from build123d import *

# Parameters (mm, degrees)
BOSS_EXTRUDE1_DEPTH = 25
SKETCH5_R           = 5
CUT_EXTRUDE1_DEPTH  = 5000
SKETCH6_R           = 5
CUT_EXTRUDE2_DEPTH  = 5000
FILLET2_R           = 10


with BuildPart() as part:
    # Sketch4 → Boss-Extrude1 (new body)
    with BuildSketch(Plane.XY):
        with BuildLine():
            ThreePointArc((0, -25), (-77.42819254, 7.07180746), (-109.5, 84.5))
            Line((-109.5, 84.5), (-109.5, -25))
            Line((-109.5, -25), (0, -25))
        make_face()
        with BuildLine():
            ThreePointArc((84.5, 84.5), (59.75052301, 24.74947699), (0, 0))
            ThreePointArc((0, 0), (-59.75052301, 24.74947699), (-84.5, 84.5))
            Line((-84.5, 84.5), (-109.5, 84.5))
            ThreePointArc((-109.5, 84.5), (-77.42819254, 7.07180746), (0, -25))
            ThreePointArc((0, -25), (77.42819254, 7.07180746), (109.5, 84.5))
            Line((109.5, 84.5), (84.5, 84.5))
        make_face()
        with BuildLine():
            Line((109.5, -25), (109.5, 84.5))
            ThreePointArc((109.5, 84.5), (77.42819254, 7.07180746), (0, -25))
            Line((0, -25), (109.5, -25))
        make_face()
    extrude(amount=BOSS_EXTRUDE1_DEPTH)

    # Sketch5 → Cut-Extrude1 (cut)
    with BuildSketch(Plane(origin=(0, 84.5, 0), x_dir=(1, 0, 0), z_dir=(0, 1, 0))):
        with Locations((-97, -12.5)):
            Circle(SKETCH5_R)
        with Locations((97, -12.5)):
            Circle(SKETCH5_R)
    extrude(amount=-CUT_EXTRUDE1_DEPTH, mode=Mode.SUBTRACT)

    # Sketch6 → Cut-Extrude2 (cut)
    with BuildSketch(Plane.XY.offset(25)):
        with Locations((-76.015, -4)):
            Circle(SKETCH6_R)
        with Locations((76.015, -4)):
            Circle(SKETCH6_R)
    extrude(amount=-CUT_EXTRUDE2_DEPTH, mode=Mode.SUBTRACT)

    # Fillet2
    fillet2_edges = [part.edges().sort_by_distance(p)[0] for p in [
        (109.5, 29.75, 25),
        (-109.5, 29.75, 25),
        (-109.5, 29.75, 0),
        (109.5, 29.75, 0),
    ]]
    fillet(fillet2_edges, radius=FILLET2_R)


solid = part.part
Could you check a few things on this model? Use its own coordinates, in mm. Give positions to 0.01 mm unless a question says otherwise; leave off trailing zeros. Order: outer loops, then holes, each group sorted by start corner. A loop starts at its lowest first (then second) coordinate and runs counter-clockwise, first axis right, second up.
1. Thinking about a two-plate mould opening in Z: for faces 1 (the flat face through (-1, -6, 0)), 2 (the flat face through (-109.5, 31, 12)), 3 (the cylindrical face through (101.619, 30.516, 14.415)), which applies, +Z half, -Z half, draft (parallel to the pull), parting line (faces both ways), or undercut?
Answers below:
face 1: -Z half
face 2: draft
face 3: undercut
2. Suppose I cut it at D-D (y = 42.5). Write out the boundary of the cut face in (x, z).
Answers below:
outline: (-109.5, 10) arc R10 ccw to (-99.5, 0) - (-73.32, 0) - (-73.32, 25) - (-99.5, 25) arc R10 ccw to (-109.5, 15) - close; (73.32, 0) - (99.5, 0) arc R10 ccw to (109.5, 10) - (109.5, 15) arc R10 ccw to (99.5, 25) - (73.32, 25) - close; hole circle Ø10 at (-97, 12.5); hole circle Ø10 at (97, 12.5)
3. I need wall thicknesses on L1, parallel to Z at x = 97, y = 27; L2, parallel to X at y = 68, z = 13.5; L3, parallel to X at y = 29.5, z = 9. Which ranges of each line are inside material? Lowest first, please.
Answers below:
L1: z = 0 to 7.5, 17.5 to 25
L2: x = -109.5 to -101.9, -92.1 to -82.87, 82.87 to 92.1, 101.9 to 109.5
L3: x = -109.45 to -100.57, -93.43 to -64.15, 64.15 to 93.43, 100.57 to 109.45
4. For pin 1 (2 mm diameter, centred on y = -4.5, z = 22, fed in from -X); pin 2 (8 mm diameter, centred on x = 97, z = 12.5, fed in from +Y); pin 3 (2 mm diameter, centred on x = 28.5, z = 15, fed in from +Y), each with a flat end and sliding along its axis, tell me the tip position at first contact or that it passes through.
Answers below:
pin 1: stops at x = -107.5
pin 2: passes through
pin 3: stops at y = 5.32
5. Suppose I cut it at C-C (x = -97). Write out the boundary of the cut face in (y, z), plus the area to 3 significant figures.
Answers below:
outline: (-25, 0) - (84.5, 0) - (84.5, 7.5) - (-25, 7.5) - close; (-25, 17.5) - (84.5, 17.5) - (84.5, 25) - (-25, 25) - close
area: 1,640 mm2
6. Suppose I cut it at A-A (y = -4). Write out the boundary of the cut face in (x, z) (3 decimals), plus the area to 3 significant figures.
Answers below:
outline: (-109.5, 10) arc R10 ccw to (-99.5, 0) - (-81.015, 0) - (-81.015, 25) - (-99.5, 25) arc R10 ccw to (-109.5, 15) - close; (-71.015, 0) - (71.015, 0) - (71.015, 25) - (-71.015, 25) - close; (81.015, 0) - (99.5, 0) arc R10 ccw to (109.5, 10) - (109.5, 15) arc R10 ccw to (99.5, 25) - (81.015, 25) - close; hole circle Ø10 at (-97, 12.5); hole circle Ø10 at (97, 12.5)
area: 4,730 mm2
7. Suppose I cut it at B-B (z = 12.5). Write out the boundary of the cut face in (x, y) (3 decimals).
Answers below:
outline: (-109.5, -25) - (-102, -25) - (-102, 84.5) - (-109.5, 84.5) - close; (-92, -25) - (92, -25) - (92, 84.5) - (84.5, 84.5) arc R84.5 cw to (-84.5, 84.5) - (-92, 84.5) - close; (102, -25) - (109.5, -25) - (109.5, 84.5) - (102, 84.5) - close; hole circle Ø10 at (-76.015, -4); hole circle Ø10 at (76.015, -4)
